The drawing under review shows one solid part. Ordinate dimensions are in mm from its lowest x, y, z. Give positions to 0.01 mm unless a question says otherwise; leave off trailing zeros. Write each loop counter-clockwise with the first axis right and the second up, starting at its lowest first coordinate (ties: lowest second). Pieces come first, ordered by that corner, then holes. Notation, with made-up numbers: (46.25, 84.25) -> (82.25, 84.25) arc R16 cw to (82.25, 103.25) -> close; hole circle Ø6 at (62, 51.5). An arc over 180 degrees is marked (long way). Use CSV: the item, a comma, the result in double quotes.
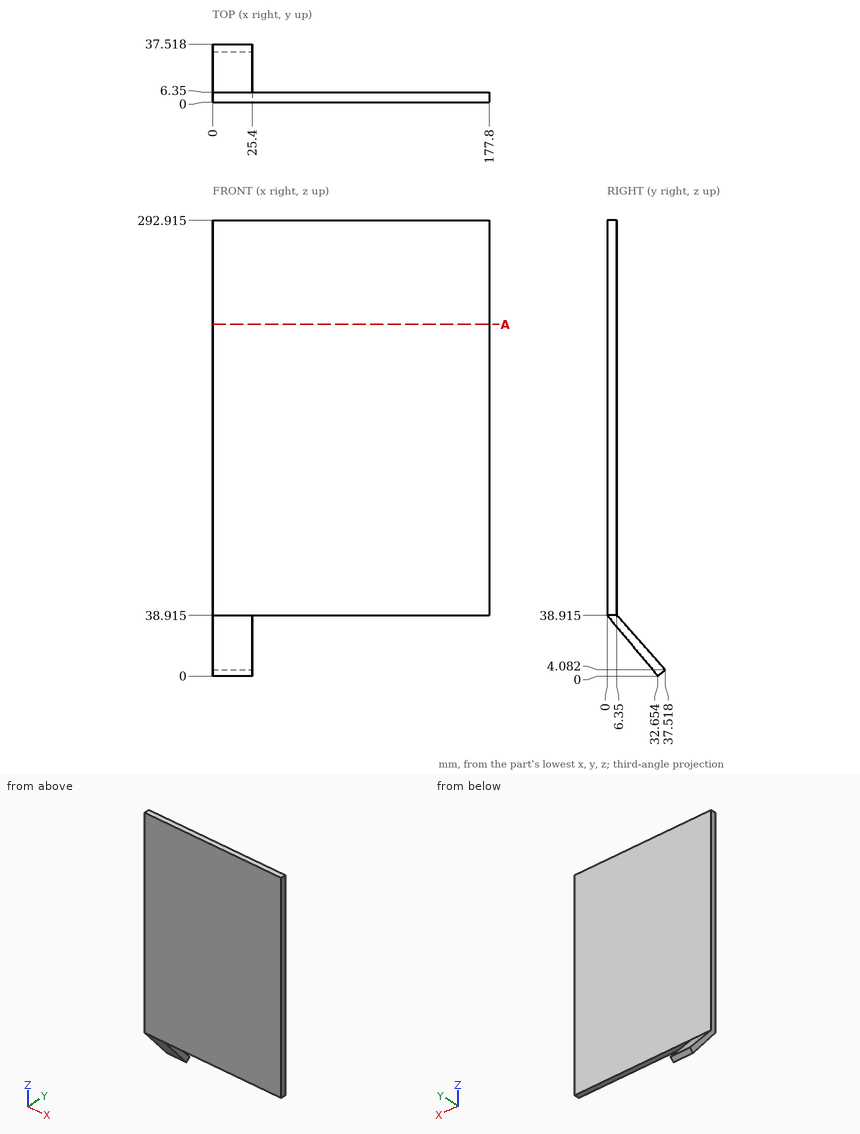
(1) Clearance check with flat-ended pins moving along their axes: pin 1 (7 mm diameter, centred on x = 76, y = 3, fed in from -Z) (1 decimal); pin 2 (5 mm diameter, centred on x = 66.5, z = 206.5, fed in from +Y); pin 3 (11.5 mm diameter, centred on y = 13, z = 24.5, fed in from +X). State where each tip first meets the part, or that it passes through.
Established:
pin 1,"stops at z = 38.9"
pin 2,"stops at y = 6.35"
pin 3,"stops at x = 25.4"
(2) For line 1 along Z through (x, y) = (83.5, 5) (1 decimal); line 2 along Y through (x, z) = (120.5, 121); line 3 along Z through (x, y) = (24, 10) (1 decimal), list the stretches that pass through material, from the lowest coordinate up. Write a range as [from, to].
Established:
line 1,"z = [38.9, 292.9]"
line 2,"y = [0, 6.35]"
line 3,"z = [27, 34.8]"
(3) Take a section at A-A (z = 226). Write out the cut boundary in (x, y), then the cut area to 3 significant figures.
Established:
outline,"(0, 0) -> (177.8, 0) -> (177.8, 6.35) -> (0, 6.35) -> close"
area,"1,130 mm2"
